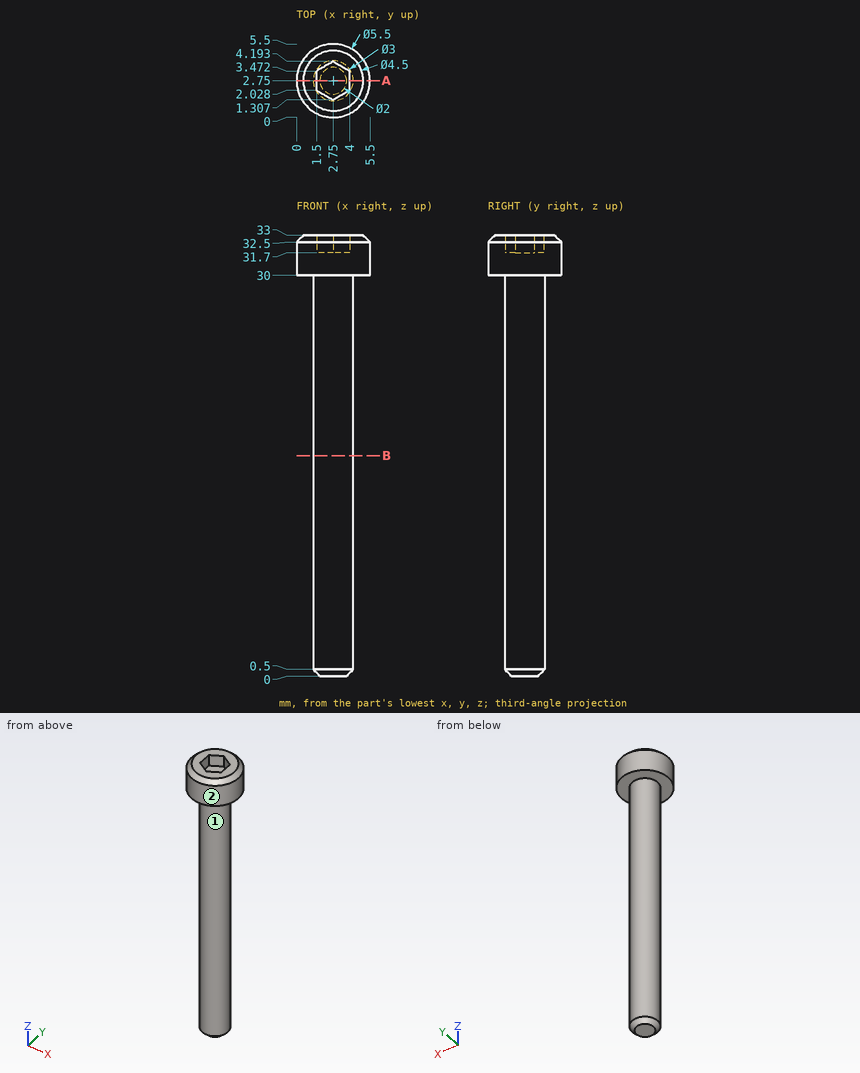
Design review of the part shown in the three views and the two pictorial views. Dimensions are in mm from the part's minimum x, y and z. A direction names the side the tool comes from. Coordinates: 2 decimals unless noted, no trailing zeros. Loops run counter-clockwise (first coordinate to the right, second up) from the corner with the lowest first, then second, coordinate; pieces in that order, holes last. Notation, with made-up numbers: (-1.75, -38) -> (46.25, -38) arc R22 ccw to (46.25, -1) -> close; hole circle Ø9 at (85, 88.5). An arc over 180 degrees is marked (long way). Answer as CSV lines item,"result".
Item 1: Insertion check: pin 1 (0.7 mm diameter, centred on y = 3, z = 32.5, fed in from -X); pin 2 (2 mm diameter, centred on x = 4.5, z = 6.5, fed in from -Y); pin 3 (1.5 mm diameter, centred on x = 2.5, z = 16.5, fed in from +Y); pin 4 (0.8 mm diameter, centred on x = 2, y = 2.5, fed in from +Z). Each pin has a flat end and moves straight along its axis. Give the tip position at first contact, or say it passes through.
Results below:
pin 1,"stops at x = 0"
pin 2,"stops at y = 1.45"
pin 3,"stops at y = 4.25"
pin 4,"stops at z = 31.7"
Item 2: Machinability: for the marked faces 1 and 2, which of the approach directions +Z, -Z, +X, -X, +Y, -Y give a long, thin tool a straight path to every point of the face, cutting with its end or side? Answer none if there is none.
Results below:
face 1,"-Z"
face 2,"+Z, -Z"
Item 3: For L1, parallel to Z at x = 2.45, y = 0.95; L2, parallel to Z at x = 3, y = 3; L3, parallel to Y at x = 4.85, z = 31 (1 decimal), list the stretches that pass through material, from the lowest coordinate up.
Results below:
L1,"z = 30 to 33"
L2,"z = 0 to 31.7"
L3,"y = 1 to 4.5"
Item 4: Take a section at B-B, the plane z = 16.5. State the section outline as (x, y) points.
Results below:
outline,"circle Ø3 at (2.75, 2.75)"
Item 5: Take a section at A-A, the plane y = 2.75. State the section outline as (x, z) points, and give its area (3 significant figures).
Results below:
outline,"(0, 30) -> (1.25, 30) -> (1.25, 0.5) -> (1.75, 0) -> (3.75, 0) -> (4.25, 0.5) -> (4.25, 30) -> (5.5, 30) -> (5.5, 32.5) -> (5, 33) -> (4, 33) -> (4, 31.7) -> (1.5, 31.7) -> (1.5, 33) -> (0.5, 33) -> (0, 32.5) -> close"
area,"103 mm2"
